Model file for the job. Use its own axes, mm. Round coordinates to 2 decimals unless told otherwise and drop trailing zeros. Order: outer loops, then holes, each group sorted by start corner. A loop starts at its lowest first (then second) coordinate and runs counter-clockwise, first axis right, second up. Notation, with made-up numbers: (62, 62.5) - (71, 62.5) arc R21 ccw to (71, 78.5) - close; hole circle Ø7 at (-17, 56.25). An arc over 180 degrees is marked (long way). Write item = value, one per line.
```python
from build123d import *

# Parameters (mm, degrees)
F2_R     = 2.5
F3_DEPTH = 11.3
F4_R     = 0.6


with BuildPart() as f1:
    # F0 (on Front) → F1 (revolve)
    with BuildSketch(Plane.XZ):
        Polygon((-4, 0), (0, 0), (0, 5), (-9.5, 5), (-9.5, 1), (-4, 1), align=None)
    revolve(axis=Axis((0, 0, 2.5), (0, 0, -1)))

    # F2 (on face) → F3 (cut)
    with BuildSketch(Plane.XY.offset(5)):
        Circle(F2_R)
    extrude(amount=-F3_DEPTH, mode=Mode.SUBTRACT)

    # F4
    f4_edges = [f1.edges().sort_by_distance(p)[0] for p in [
        (9.5, 0, 5),
        (9.5, 0, 1),
        (4, 0, 1),
    ]]
    fillet(f4_edges, radius=F4_R)


solid = f1.part
```
1) Flat gauge pins, fed straight in: pin 1 Ø3 at (x, y) = (-7, -3) entering from -Z; pin 2 Ø4.5 at (x, y) = (0, 0) entering from +Z; pin 3 Ø3 at (y, z) = (-5, 3.5) entering from +X; pin 4 Ø2 at (x, z) = (5, 4) entering from +Y. Where does each tip first touch, or does it go through?
Conclusion:
pin_1 = 1
pin_2 = through
pin_3 = 8.83
pin_4 = 8.62
2) Wall check: line 1 along Y through (x, z) = (0, 2.1); line 2 along Z through (x, y) = (4, 2.5); line 3 along Y through (x, z) = (-1, 3). Give the ranges that are in metal, low to high.
Conclusion:
line_1 = -9.5 to -2.5, 2.5 to 9.5
line_2 = 1 to 5
line_3 = -9.45 to -2.29, 2.29 to 9.45
3) Mould opens along X. For faces 1 (the face through (-4, -4, 1)), 2 (the face through (0.867, -3.905, 0.197)), 3 (the face through (-0.54, -2.44, 2.54)) say: +X half, -X half, draft (parallel to the pull), parting line (faces both ways), or undercut.
Conclusion:
face_1 = draft
face_2 = parting line
face_3 = undercut
4) Cut at A-A (y = 0). Write the cut outline in (x, z).
Conclusion:
outline = (-9.5, 1.6) arc R0.6 ccw to (-8.9, 1) - (-4.6, 1) arc R0.6 cw to (-4, 0.4) - (-4, 0) - (-2.5, 0) - (-2.5, 5) - (-8.9, 5) arc R0.6 ccw to (-9.5, 4.4) - close; (2.5, 0) - (4, 0) - (4, 0.4) arc R0.6 cw to (4.6, 1) - (8.9, 1) arc R0.6 ccw to (9.5, 1.6) - (9.5, 4.4) arc R0.6 ccw to (8.9, 5) - (2.5, 5) - close
5) Cut at C-C (z = 2.65). Write the cut outline in (x, y).
Conclusion:
outline = circle Ø19 at (0, 0); hole circle Ø5 at (0, 0)
